```python
from build123d import *

# Parameters (mm, degrees)
F0_R            = 53.975
F0_R_2          = 20.32
F1_DEPTH        = 6.35
F2_D            = 4.7625
F2_DEPTH        = 6.35
F2_TIP          = 1.4307993491
F2_COPIES_COUNT = 6


# Not quite as in the source:
# - a pattern or mirror of a feature is missing from the dataset's text; its kind, count and spacing are read off the source's solid


with BuildPart() as f1:
    # F0 (on Top) → F1 (new body)
    with BuildSketch(Plane.XY):
        Circle(F0_R)
        Circle(F0_R_2, mode=Mode.SUBTRACT)
    extrude(amount=F1_DEPTH)

    # F2
    with Locations(Plane(origin=(0, 0, 0), x_dir=(1, 0, 0), z_dir=(0, 0, -1))):
        with Locations((0, 25.4)):
            f2 = Hole(F2_D / 2, depth=F2_DEPTH)
            with Locations((0, 0, -(F2_DEPTH + F2_TIP / 2))):  # 118° drill point
                Cone(0, F2_D / 2, F2_TIP, mode=Mode.SUBTRACT)

    # F2_copies: F2 ×6 about axis
    f2_copies_axis = Axis((0, 0, 0), (0, 0, 1))
    for i in range(1, F2_COPIES_COUNT):
        add(f2.rotate(f2_copies_axis, i * 360 / F2_COPIES_COUNT), mode=Mode.SUBTRACT)


solid = f1.part
```
Here's how the part is built. I have some questions about the finished solid (model axes, mm). Round coordinates to 2 decimals unless told otherwise and drop trailing zeros. Write each loop counter-clockwise with the first axis right and the second up, starting at its lowest first coordinate (ties: lowest second). Pieces come first, ordered by that corner, then holes.
Q1. If we mould it in two halves opening along Y, with no side actions, what happens to faces 1 (the cylindrical face through (1.755, -27.009, 3.219)), 2 (the cylindrical face through (-39.78, 36.48, 3.13)), 3 (the flat face through (23, 1, 6.35)), 4 (the cylindrical face through (24.376, 12.595, 3.219))? For each: +Y half, -Y half, draft (parallel to the pull), parting line (faces both ways), or undercut.
Q2. If we section it at D-D on y = -12.7: Write out the boundary of the cut face in (x, z).
Q3. If we section it at C-C on z = 4: Give the number of separate pieces and of enclosed holes in the cut face, plus the area to 3 significant figures.
Q4. If we section it at A-A on y = 0: Write out the boundary of the cut face in (x, z) (3 decimals), plus the area to 3 significant figures.
Q5. Will these pins go through, and if not, where does the flat tip stop? P1, Ø4.5, axis at x = 22, y = 12.7, coming from the -Z side; P2, Ø5.5, axis at x = 0, y = 25.4, coming from the -Z side; P3, Ø2, axis at y = -42.5, z = 2, coming from the +X side; P4, Ø3, axis at y = 17, z = 2.5, coming from the -X side.
Q6. If we section it at B-B on x = 9.5: Write out the boundary of the cut face in (y, z).
Q7. Please list where these lines run through material, in increasing order: probe 1 along Y at (x, z) = (0, 2) (3 decimals); probe 2 along Y at (x, z) = (-1, 2); probe 3 along X at (y, z) = (-12.7, 3.75).
Answer below:
1. face 1: undercut
1. face 2: parting line
1. face 3: draft
1. face 4: undercut
2. outline: (-52.46, 0) - (-24.38, 0) - (-24.38, 6.35) - (-52.46, 6.35) - close; (-19.62, 0) - (-15.86, 0) - (-15.86, 6.35) - (-19.62, 6.35) - close; (15.86, 0) - (19.62, 0) - (19.62, 6.35) - (15.86, 6.35) - close; (24.38, 0) - (52.46, 0) - (52.46, 6.35) - (24.38, 6.35) - close
3. separate pieces: 1
3. enclosed holes: 7
3. area: 7,750 mm2
4. outline: (-53.975, 0) - (-20.32, 0) - (-20.32, 6.35) - (-53.975, 6.35) - close; (20.32, 0) - (53.975, 0) - (53.975, 6.35) - (20.32, 6.35) - close
4. area: 427 mm2
5. P1: passes through
5. P2: stops at z = 0
5. P3: stops at x = 34.51
5. P4: stops at x = -51.7
6. outline: (-53.13, 0) - (-17.96, 0) - (-17.96, 6.35) - (-53.13, 6.35) - close; (17.96, 0) - (53.13, 0) - (53.13, 6.35) - (17.96, 6.35) - close
7. probe 1: y = -53.975 to -27.781, -23.019 to -20.32, 20.32 to 23.019, 27.781 to 53.975
7. probe 2: y = -53.97 to -27.56, -23.24 to -20.3, 20.3 to 23.24, 27.56 to 53.97
7. probe 3: x = -52.46 to -24.38, -19.62 to -15.86, 15.86 to 19.62, 24.38 to 52.46
